Autodesk Inventor part; units mm, degrees
ref_plane "YZ Plane" through (0, 0, 0) normal (1, 0, 0) x (0, 1, 0)
ref_plane "XZ Plane" through (0, 0, 0) normal (0, 1, 0) x (-1, 0, 0)
ref_plane "XY Plane" through (0, 0, 0) normal (0, 0, 1) x (1, 0, 0)
sketch "Эскиз1" plane through (0, 0, 0) normal (0, 0, 1) x (1, 0, 0)
  circle A0 centre (0, 0) radius 6
  dimension "d0" = 12
extrude "Выдавливание1" add sketch "Эскиз1" along normal blind 55
sketch "Эскиз2" plane through (0, 0, 55) normal (0, 0, 1) x (1, 0, 0)
  circle A0 centre (0, 0) radius 5.25
  dimension "d3" = 10.5
extrude "Выдавливание2" add sketch "Эскиз2" along normal blind 8
sketch "Эскиз3" plane through (0, 0, 0) normal (0, 0, -1) x (-1, 0, 0)
  circle A0 centre (0, 0) radius 5.25
  dimension "d6" = 10.5
extrude "Выдавливание3" add sketch "Эскиз3" along normal blind 1
thread "Резьба1"
sketch "Эскиз4" plane through (0, 0, -1) normal (0, 0, -1) x (-1, 0, 0)
  circle A0 centre (0, 2) radius 2.75
  circle A1 centre (0, 2) radius 2.5
  point P0 (0, 0)
  dimension "d11" = 5.5
  dimension "d12" = 2
  dimension "d13" = 5
extrude "Выдавливание4" add sketch "Эскиз4" along normal blind 5
sketch "Эскиз5" plane through (0, 0, -1) normal (0, 0, -1) x (-1, 0, 0)
  circle A0 centre (0, -3) radius 1.5
  point P0 (0, 0)
  dimension "d16" = 3
  dimension "d17" = 3
extrude "Выдавливание5" add sketch "Эскиз5" along normal blind 1
fillet "Сопряжение1" radius 1 1 edges at (1.5, -3, -2)
properties part number "LJ12A3-4-Z-BX"
Geometry: final body of the model. Coordinates: model frame, mm. A direction names the side the tool comes from. Coordinates: 2 decimals unless noted, no trailing zeros. Order: outer loops, then holes, each group sorted by start corner. A loop starts at its lowest first (then second) coordinate and runs counter-clockwise, first axis right, second up. Notation, with made-up numbers: (87, 4.5) -> (92, 4.5) arc R9 ccw to (92, 17.5) -> close; hole circle Ø7 at (16, 60). An arc over 180 degrees is marked (long way). Answer in a Markdown table with one row per item.
Item 1: Access query for faces 4 (the cylindrical face through (-6, 0, 27)), 5 (the flat face through (0, 2, -1)), 6 (the cylindrical face through (5, -1.6, 58.9)). Directions: +Z, -Z, +X, -X, +Y, -Y. A direction counts if a zero-diameter tool reaches every point of the face in a straight line with its end or side. Return the directions, or none.
Return value:
| item | result |
|---|---|
| face 4 | +Z, -Z |
| face 5 | -Z |
| face 6 | +Z |
Item 2: Draft query along Y for faces 1 (the cylindrical face through (-1.15, 4.22, -3.46)), 2 (the cylindrical face through (-5, -1.6, -0.5)), 3 (the flat face through (4, -4, 55)). Return one class per face: released by +Y, released by -Y, zero draft, split by the parting line, or undercut.
Return value:
| item | result |
|---|---|
| face 1 | undercut |
| face 2 | split by the parting line |
| face 3 | zero draft |
Item 3: Contact query for flat-ended pins moving along their axis: P1, Ø3, axis at x = 0, y = 1.5, coming from the -Z side; P2, Ø2, axis at x = 2.5, z = 49, coming from the -Y side; P3, Ø2, axis at y = 3, z = 48.5, coming from the +X side. Output: stop coordinate, or through.
Return value:
| item | result |
|---|---|
| P1 | stops at z = -1 |
| P2 | stops at y = -5.81 |
| P3 | stops at x = 5.66 |
Item 4: Section B-B on z = 58.5. Output: boundary loops of the cut face in (x, y), plus the area to 3 significant figures.
Return value:
| item | result |
|---|---|
| outline | circle Ø10.5 at (0, 0) |
| area | 86.6 mm² |
Item 5: Ray query, L1, parallel to Y at x = 0, z = -3.7; L2, parallel to Z at x = 0.75, y = 5; L3, parallel to Z at x = -4.25, y = -3.75. Return the intervals inside material, ascending.
Return value:
| item | result |
|---|---|
| L1 | y = -0.75 to -0.5, 4.5 to 4.75 |
| L2 | z = -1 to 63 |
| L3 | z = 0 to 55 |
Item 6: Section A-A on y = 2. Output: boundary loops of the cut face in (x, z).
Return value:
| item | result |
|---|---|
| outline | (-5.66, 0) -> (-4.85, 0) -> (-4.85, -1) -> (-2.75, -1) -> (-2.75, -6) -> (-2.5, -6) -> (-2.5, -1) -> (2.5, -1) -> (2.5, -6) -> (2.75, -6) -> (2.75, -1) -> (4.85, -1) -> (4.85, 0) -> (5.66, 0) -> (5.66, 55) -> (4.85, 55) -> (4.85, 63) -> (-4.85, 63) -> (-4.85, 55) -> (-5.66, 55) -> close |
Item 7: Section C-C on z = 21. Output: boundary loops of the cut face in (x, y), plus the area to 3 significant figures.
Return value:
| item | result |
|---|---|
| outline | circle Ø12 at (0, 0) |
| area | 113 mm² |
